Source: CAD feature listing. Evaluate the final solid. Frame: model axes, mm. Face numbers are marked on the shaded views. A direction names the side the tool comes from. Coordinates: 2 decimals unless noted, no trailing zeros. Write each loop counter-clockwise with the first axis right and the second up, starting at its lowest first coordinate (ties: lowest second). Pieces come first, ordered by that corner, then holes. Notation, with made-up numbers: (-21.5, 17) - (4.5, 17) arc R22 ccw to (4.5, 40) - close; hole circle Ø7 at (15, 11). An arc over 180 degrees is marked (long way). One line per item, written item: value.
from build123d import *

# Parameters (mm, degrees)
F0_W          = 3.81
F0_H          = 38.1
F1_DEPTH      = 3.81
F2_R          = 2.8295085799
F3_DEPTH      = 19.05
F3_DEPTH_BACK = 19.05
F4_R          = 1.905
F5_DEPTH      = 47.01882
F6_W          = 11.7936587512
F6_H          = 46.736
F7_DEPTH      = 14.81339
F8_W          = 8.9291655459
F8_H          = 39.4763015211
F9_DEPTH      = 25.4
F10_T1_DEPTH  = 11.7936587512
F10_T3_DEPTH  = 11.7936587512
F10_T5_DEPTH  = 11.7936587512
F10_T7_DEPTH  = 11.7936587512
F10_T9_DEPTH  = 39.4763015211
F10_T11_DEPTH = 37.1936587512
F10_T13_DEPTH = 37.1936587512
F10_T15_DEPTH = 39.4763015211
F11_T1_DEPTH  = 75.3934442484
F11_T3_DEPTH  = 31.3467221242
F11_T5_DEPTH  = 31.3467221242
F11_T7_DEPTH  = 49.1322772947
F11_T9_DEPTH  = 51.6998748204


# Not quite as in the source:
# - a fillet or chamfer that OpenCascade refuses, or shapes differently, is made with other operations: its cross-section is extruded or revolved along the edge and cut away or added


with BuildPart() as f1:
    # F0 (on Front) → F1 (new body)
    with BuildSketch(Plane.XZ):
        Polygon((0, 38.1), (-50.8, 38.1), (-50.8, -38.1), (0, -38.1), (0, -19.05), (0, 19.05), align=None)
        with Locations((1.905, 0)):
            Rectangle(F0_W, F0_H)
    extrude(amount=F1_DEPTH)

    # F2 (on Top) → F3 (join, two sides)
    with BuildSketch(Plane.XY) as f3_sk:
        with Locations((6.3444059342, -1.762334723)):
            Circle(F2_R)
    extrude(amount=F3_DEPTH)
    extrude(f3_sk.sketch, amount=-F3_DEPTH_BACK)

    # F4 (on face) → F5 (cut)
    with BuildSketch(Plane.XY.offset(19.05)):
        with Locations((6.3444059342, -1.762334723)):
            Circle(F4_R)
    extrude(amount=-F5_DEPTH, mode=Mode.SUBTRACT)

    # F6 (on face) → F7 (join)
    with BuildSketch(Plane(origin=(0, 0, 0), x_dir=(-1, 0, 0), z_dir=(0, 1, 0))):
        with Locations((44.9031706244, 0)):
            Rectangle(F6_W, F6_H)
    extrude(amount=F7_DEPTH)

    # F8 (on face) → F9 (cut)
    with BuildSketch(Plane(origin=(-50.8, 0, 0), x_dir=(0, -1, 0), z_dir=(-1, 0, 0))):
        with Locations((-6.8143603858, -0.5874447525)):
            Rectangle(F8_W, F8_H)
    extrude(amount=-F9_DEPTH, mode=Mode.SUBTRACT)

    # F10: fillet of radius 5.08 on 8 edges, made by hand

    # F10_s2 → F10_t1 (join)
    with BuildSketch(Plane.YZ.offset(-50.8)):
        with BuildLine():
            ThreePointArc((0, -28.448), (1.4878975516, -24.8558975516), (5.08, -23.368))
            Line((5.08, -23.368), (0, -23.368))
            Line((0, -23.368), (0, -28.448))
        make_face()
    extrude(amount=F10_T1_DEPTH)

    # F10_s4 → F10_t3 (join)
    with BuildSketch(Plane.YZ.offset(-50.8)):
        with BuildLine():
            ThreePointArc((0, 28.448), (1.4878975516, 24.8558975516), (5.08, 23.368))
            Line((5.08, 23.368), (0, 23.368))
            Line((0, 23.368), (0, 28.448))
        make_face()
    extrude(amount=F10_T3_DEPTH)

    # F10_s6 → F10_t5 (join)
    with BuildSketch(Plane.YZ.offset(-50.8)):
        with BuildLine():
            ThreePointArc((11.2789431587, -15.245595513), (9.7910456071, -18.8376979614), (6.1989431587, -20.325595513))
            Line((6.1989431587, -20.325595513), (11.2789431587, -20.325595513))
            Line((11.2789431587, -20.325595513), (11.2789431587, -15.245595513))
        make_face()
    extrude(amount=F10_T5_DEPTH)

    # F10_s8 → F10_t7 (join)
    with BuildSketch(Plane.YZ.offset(-50.8)):
        with BuildLine():
            ThreePointArc((6.1989431587, 19.1507060081), (9.7910456071, 17.6628084565), (11.2789431587, 14.0707060081))
            Line((11.2789431587, 14.0707060081), (11.2789431587, 19.1507060081))
            Line((11.2789431587, 19.1507060081), (6.1989431587, 19.1507060081))
        make_face()
    extrude(amount=F10_T7_DEPTH)

    # F10_s10 → F10_t9 (cut)
    with BuildSketch(Plane.XY.offset(-20.325595513)):
        with BuildLine():
            ThreePointArc((-50.8, -2.7302223872), (-49.3121024484, 0.8618800613), (-45.72, 2.3497776128))
            Line((-45.72, 2.3497776128), (-50.8, 2.3497776128))
            Line((-50.8, 2.3497776128), (-50.8, -2.7302223872))
        make_face()
    extrude(amount=F10_T9_DEPTH, mode=Mode.SUBTRACT)

    # F10_s12 → F10_t11 (cut)
    with BuildSketch(Plane.YZ.offset(-63.5)):
        with BuildLine():
            ThreePointArc((14.81339, 18.288), (13.3254924484, 21.8801024484), (9.73339, 23.368))
            Line((9.73339, 23.368), (14.81339, 23.368))
            Line((14.81339, 23.368), (14.81339, 18.288))
        make_face()
    extrude(amount=F10_T11_DEPTH, mode=Mode.SUBTRACT)

    # F10_s14 → F10_t13 (cut)
    with BuildSketch(Plane.YZ.offset(-63.5)):
        with BuildLine():
            ThreePointArc((14.81339, -18.288), (13.3254924484, -21.8801024484), (9.73339, -23.368))
            Line((9.73339, -23.368), (14.81339, -23.368))
            Line((14.81339, -23.368), (14.81339, -18.288))
        make_face()
    extrude(amount=F10_T13_DEPTH, mode=Mode.SUBTRACT)

    # F10_s16 → F10_t15 (cut)
    with BuildSketch(Plane.XY.offset(-20.325595513)):
        with BuildLine():
            ThreePointArc((-39.0063412488, 0), (-40.8472599359, 1.7237606464), (-43.2902980315, 2.3497776128))
            Line((-43.2902980315, 2.3497776128), (-39.0063412488, 2.3497776128))
            Line((-39.0063412488, 2.3497776128), (-39.0063412488, 0))
        make_face()
    extrude(amount=F10_T15_DEPTH, mode=Mode.SUBTRACT)

    # F11: fillet of radius 5.08 on 6 edges, made by hand

    # F11_s2 → F11_t1 (cut)
    with BuildSketch(Plane.YZ.offset(-63.0967221242)):
        with BuildLine():
            ThreePointArc((0, -33.1813111503), (-1.0639073716, -36.2921631237), (-3.81, -38.1))
            Line((-3.81, -38.1), (0, -38.1))
            Line((0, -38.1), (0, -33.1813111503))
        make_face()
        with BuildLine():
            ThreePointArc((-3.81, 38.1), (-1.0639073716, 36.2921631237), (0, 33.1813111503))
            Line((0, 33.1813111503), (0, 38.1))
            Line((0, 38.1), (-3.81, 38.1))
        make_face()
    extrude(amount=F11_T1_DEPTH, mode=Mode.SUBTRACT)

    # F11_s4 → F11_t3 (cut)
    with BuildSketch(Plane.XY.offset(19.05)):
        with BuildLine():
            ThreePointArc((0, -3.81), (-1.8078368763, -1.0639073716), (-4.9186888497, 0))
            Line((-4.9186888497, 0), (0, 0))
            Line((0, 0), (0, -3.81))
        make_face()
    extrude(amount=F11_T3_DEPTH, mode=Mode.SUBTRACT)

    # F11_s6 → F11_t5 (cut)
    with BuildSketch(Plane.XY.offset(-50.3967221242)):
        with BuildLine():
            ThreePointArc((-4.9186888497, 0), (-1.8078368763, -1.0639073716), (0, -3.81))
            Line((0, -3.81), (0, 0))
            Line((0, 0), (-4.9186888497, 0))
        make_face()
    extrude(amount=F11_T5_DEPTH, mode=Mode.SUBTRACT)

    # F11_s8 → F11_t7 (cut)
    with BuildSketch(Plane.XY.offset(-24.5661386473)):
        with BuildLine():
            ThreePointArc((1.6035445411, 0), (2.7352095066, -0.1276536464), (3.81, -0.5041990529))
            Line((3.81, -0.5041990529), (3.81, 0))
            Line((3.81, 0), (1.6035445411, 0))
        make_face()
    extrude(amount=F11_T7_DEPTH, mode=Mode.SUBTRACT)

    # F11_s10 → F11_t9 (cut)
    with BuildSketch(Plane.XY.offset(-25.8499374102)):
        with BuildLine():
            ThreePointArc((1.0900250359, -3.81), (2.5061483361, -3.6086263229), (3.81, -3.0204703932))
            Line((3.81, -3.0204703932), (3.81, -3.81))
            Line((3.81, -3.81), (1.0900250359, -3.81))
        make_face()
    extrude(amount=F11_T9_DEPTH, mode=Mode.SUBTRACT)


solid = f1.part
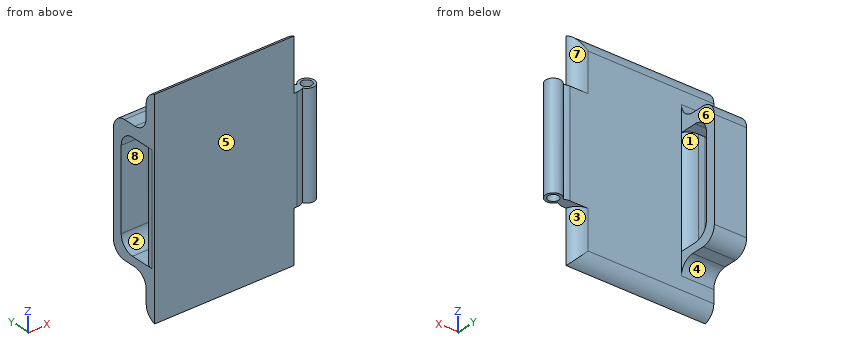
1) Draft query along X for the marked faces 1, 2 and 3. Return one class per face: released by +X, released by -X, zero draft, split by the parting line, or undercut.
Values found:
face 1: undercut
face 2: zero draft
face 3: released by +X
2) Section query D-D on x = -3. Output: boundary loops of the cut face in (y, z).
Values found:
outline: (-3.81, -38.1) arc R5.08 ccw to (-0.38, -35.1) - (-0.38, -19.05) - (0, -19.05) - (0, 19.05) - (-0.38, 19.05) - (-0.38, 35.1) arc R5.08 ccw to (-3.81, 38.1) - close
3) Section query C-C on y = 8.5. Output: boundary loops of the cut face in (x, z).
Values found:
outline: (-50.8, -23.37) - (-39.01, -23.37) - (-39.01, -19.77) - (-50.8, -19.77) - close; (-50.8, 18.6) - (-39.01, 18.6) - (-39.01, 23.37) - (-50.8, 23.37) - close
4) Section query B-B on x = -44.5. Output: boundary loops of the cut face in (y, z), then the cut area to 3 significant figures.
Values found:
outline: (-3.81, -38.1) arc R5.08 ccw to (0, -33.18) - (0, -28.45) arc R5.08 cw to (5.08, -23.37) - (9.73, -23.37) arc R5.08 ccw to (14.81, -18.29) - (14.81, 18.29) arc R5.08 ccw to (9.73, 23.37) - (5.08, 23.37) arc R5.08 cw to (0, 28.45) - (0, 33.18) arc R5.08 ccw to (-3.81, 38.1) - close; hole (2.35, -20.33) - (6.2, -20.33) arc R5.08 ccw to (11.28, -15.25) - (11.28, 14.07) arc R5.08 ccw to (6.2, 19.15) - (2.35, 19.15) - close
area: 632 mm2
5) Contact query for flat-ended pins moving along their axis: P1, Ø2, axis at x = -21.5, y = -1, coming from the +Z side; P2, Ø1, axis at x = -40.5, y = 11, coming from the +Z side; P3, Ø1.4, axis at x = -43.5, y = 6.5, coming from the -Z side. Output: stop coordinate, or through.
Values found:
P1: z = 37.22
P2: z = 23.31
P3: z = -23.37
6) Reachability of the marked faces 4, 5, 6, 7 and 8 from +Z, -Z, +X, -X, +Y, -Y: full face, straight path, thin tool, end or side. Return the list, or none.
Values found:
face 4: -Z, +X, -X, +Y
face 5: +Z, -Z, -X, -Y
face 6: +Z, -Z, +X, +Y
face 7: +Z, +X, +Y
face 8: +X, -X
7) Section query A-A on z = -10. Output: boundary loops of the cut face in (x, y) (1 decimal).
Values found:
outline: (-50.8, -3.8) - (1.1, -3.8) arc R5.1 ccw to (3.8, -3) arc R2.8 ccw (long way) to (3.8, -0.5) arc R5.1 ccw to (1.6, 0) - (-39, 0) arc R5.1 ccw to (-43.3, 2.3) - (-45.7, 2.3) arc R5.1 ccw to (-50.8, -2.7) - close; (-50.8, 11.3) - (-39, 11.3) - (-39, 14.8) - (-50.8, 14.8) - close; hole circle Ø3.8 at (6.3, -1.8)
8) Material intervals for line 1 (X direction, y = -2.5, z = -17); line 2 (Y direction, x = -32, z = -1.5); line 3 (Z direction, x = -2.5, y = -0.5), sorted ascending.
Values found:
line 1: -50.79 to 4.59, 8.1 to 9.08
line 2: -3.81 to 0
line 3: -19.05 to 19.05
